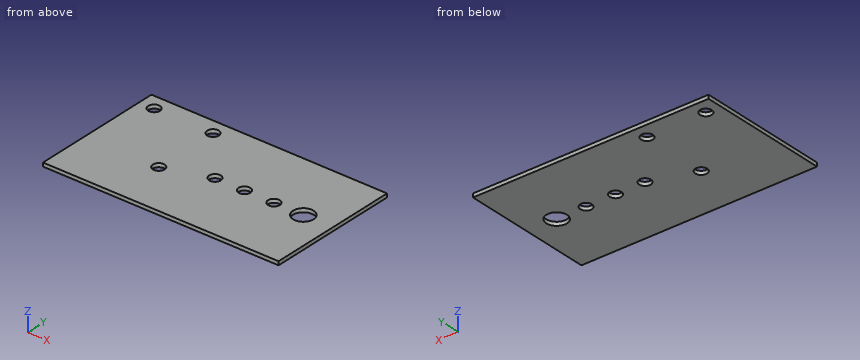
Autodesk Inventor part; units mm, degrees
ref_plane "YZ Plane" through (0, 0, 0) normal (1, 0, 0) x (0, 1, 0)
ref_plane "XZ Plane" through (0, 0, 0) normal (0, 1, 0) x (-1, 0, 0)
ref_plane "XY Plane" through (0, 0, 0) normal (0, 0, 1) x (1, 0, 0)
sketch "Sketch1" plane through (0, 0, 0) normal (0, 0, 1) x (1, 0, 0)
  line L0 (0, 0) -> (101.6, 0)
  line L1 (101.6, 0) -> (101.6, 57.15)
  line L2 (101.6, 57.15) -> (0, 57.15)
  line L3 (0, 57.15) -> (0, 0)
  line L4 (2.6205, 15.875) -> (101.6, 15.875)
  line L5 (2.6205, 15.875) -> (0, 15.875)
  circle A0 centre (88.9, 28.575) radius 4.445
  circle A1 centre (76.2, 28.575) radius 2.54
  circle A2 centre (63.5, 28.575) radius 2.54
  circle A3 centre (50.8, 28.575) radius 2.54
  circle A4 centre (31.75, 22.225) radius 2.54
  circle A5 centre (6.35, 50.8) radius 2.54
  circle A6 centre (31.75, 50.8) radius 2.54
  dimension "d0" = 101.6
  dimension "d1" = 57.15
  dimension "d7" = 8.89
  dimension "d11" = 5.08
  dimension "d12" = 5.08
  dimension "d13" = 5.08
  dimension "d16" = 5.08
  dimension "d21" = 5.08
  dimension "d23" = 5.08
extrude "Extrusion2" add sketch "Sketch1" along normal blind 1.5875
properties part number "flatPoly2ForCNC"
Here's how the part is built. I have some questions about the finished solid (model axes, mm). Coordinates: 2 decimals unless noted, no trailing zeros. Loops run counter-clockwise (first coordinate to the right, second up) from the corner with the lowest first, then second, coordinate; pieces in that order, holes last. Notation, with made-up numbers: (61.5, 48.25) -> (74.5, 48.25) arc R24 cw to (74.5, 74.25) -> close; hole circle Ø9 at (89, 25). An arc over 180 degrees is marked (long way). Use one line per item in the form item = value. Start each with the question number.
(1) If we section it at C-C (x = 31.75): Give the number of separate pieces and of enclosed holes in the cut face, then the cut area to 3 significant figures.
(2) Will this pin go through, and if not, where does the flat tip stop? pin 1 (8 mm diameter, centred on x = 31.75, y = 22.225, fed in from -Z).
(3) Please list where these lines run through material, in increasing order: line 1 along Y through (x, z) = (31.75, 1) (3 decimals); line 2 along Y through (x, z) = (50.8, 1.35) (3 decimals); line 3 along X through (y, z) = (29.5, 1.3).
(4) If we section it at B-B (y = 50.8): Please give me the cut outline in (x, z), then the cut area to 3 significant figures.
(5) If we section it at A-A (x = 88.9): Please give me the cut outline in (y, z), then the cut area to 3 significant figures.
(6) If we section it at D-D (z = 0.95): Please give me the cut outline in (x, y) (3 decimals).
Verdict:
q1.separate_pieces = 3
q1.enclosed_holes = 0
q1.area = 74.6 mm²
q2.pin_1 = 0
q3.line_1 = 0 to 19.685, 24.765 to 48.26, 53.34 to 57.15
q3.line_2 = 0 to 26.035, 31.115 to 57.15
q3.line_3 = 0 to 48.43, 53.17 to 61.13, 65.87 to 73.83, 78.57 to 84.55, 93.25 to 101.6
q4.outline = (0, 0) -> (3.81, 0) -> (3.81, 1.59) -> (0, 1.59) -> close; (8.89, 0) -> (29.21, 0) -> (29.21, 1.59) -> (8.89, 1.59) -> close; (34.29, 0) -> (101.6, 0) -> (101.6, 1.59) -> (34.29, 1.59) -> close
q4.area = 145 mm²
q5.outline = (0, 0) -> (24.13, 0) -> (24.13, 1.59) -> (0, 1.59) -> close; (33.02, 0) -> (57.15, 0) -> (57.15, 1.59) -> (33.02, 1.59) -> close
q5.area = 76.6 mm²
q6.outline = (0, 0) -> (101.6, 0) -> (101.6, 57.15) -> (0, 57.15) -> close; hole circle Ø5.08 at (6.35, 50.8); hole circle Ø5.08 at (31.75, 22.225); hole circle Ø5.08 at (31.75, 50.8); hole circle Ø5.08 at (50.8, 28.575); hole circle Ø5.08 at (63.5, 28.575); hole circle Ø5.08 at (76.2, 28.575); hole circle Ø8.89 at (88.9, 28.575)
